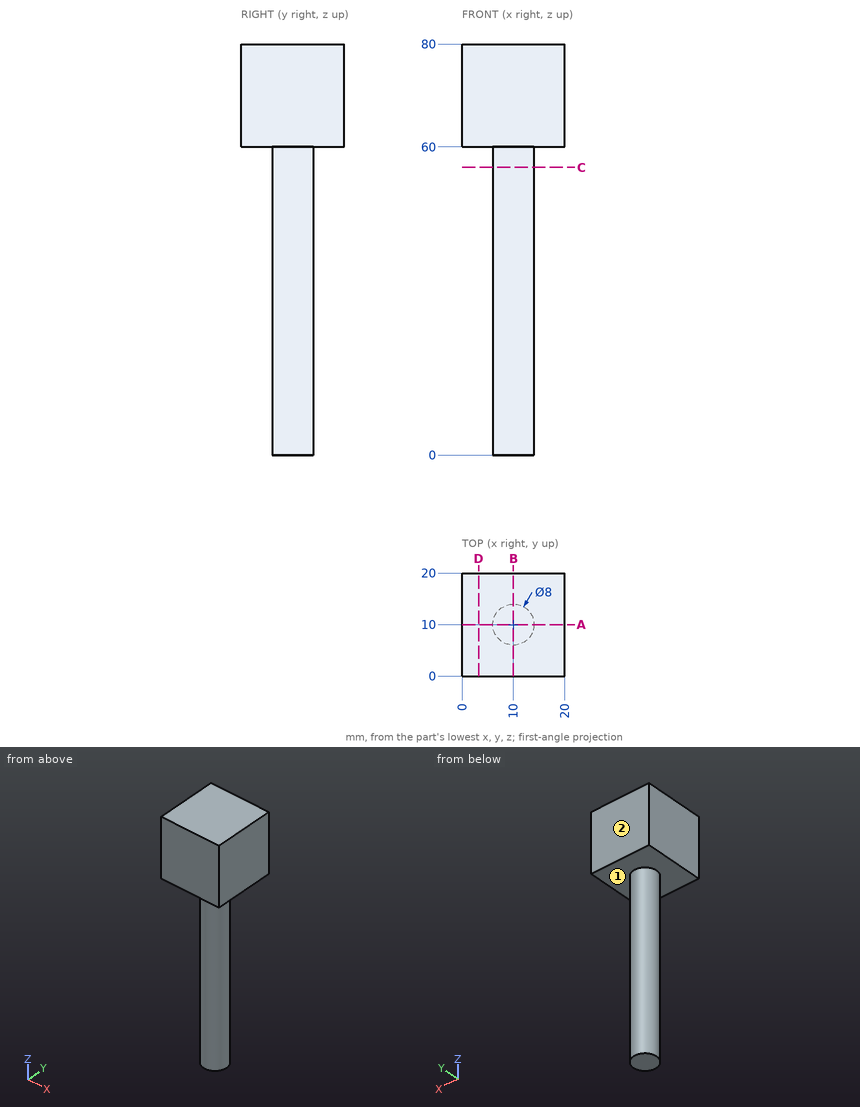
Answer from the drawing. Dimensions are ordinates in mm from the lowest x, y and z of the part. A direction names the side the tool comes from. Round coordinates to 2 decimals unless told otherwise and drop trailing zeros. Write each loop counter-clockwise with the first axis right and the second up, starting at its lowest first coordinate (ties: lowest second). Pieces come first, ordered by that corner, then holes. Notation, with made-up numbers: M -26,64 L 27,64 A19 ccw 27,94 Z; hole C 60,39.25 d11. An arc over 180 degrees is marked long. Write each question's results on one line, items separated by ' | '. Start each with the question number.
Item 1: Straight lines are drawn through the part: L1, parallel to Z at x = 11.5, y = 6.25; L2, parallel to X at y = 9.75, z = 9.5; L3, parallel to Y at x = 10, z = 14.5. For each, find the intervals that lie inside material, in ascending order. Write a range as [from, to].
Item 2: Flat-ended cylindrical pins translate along their axes: pin 1 Ø10 at (x, z) = (6.5, 53) entering from +Y; pin 2 Ø6 at (x, z) = (13, 26) entering from -Y; pin 3 Ø3 at (y, z) = (14, 43) entering from +X; pin 4 Ø4 at (y, z) = (3, 31.5) entering from -X. Find the tip coordinate at first contact, or state that the pin passes through.
Item 3: A cutting plane is placed at C-C on z = 56. Write down the section's boundary in (x, y).
Item 4: A cutting plane is placed at A-A on y = 10. Write down the section's boundary in (x, z).
Item 5: For the marked faces 1 and 2, determine the directions among +Z, -Z, +X, -X, +Y, -Y from which every point of the face is accessible in a straight line to the end or side of a thin tool.
Item 6: A cutting plane is placed at D-D on x = 3.25. Write down the section's boundary in (y, z), and give its area (3 significant figures).
Check sheet entries:
1) L1: [60, 80] | L2: [6.01, 13.99] | L3: [6, 14]
2) pin 1: y = 14 | pin 2: y = 6 | pin 3: x = 13.12 | pin 4: through
3) outline: C 10,10 d8
4) outline: M 0,60 L 6,60 L 6,0 L 14,0 L 14,60 L 20,60 L 20,80 L 0,80 Z
5) face 1: -Z | face 2: +Z, -Z, +X, -X, +Y
6) outline: M 0,60 L 20,60 L 20,80 L 0,80 Z | area: 400 mm²
